```python
from build123d import *

# Parameters (mm, degrees)
SKETCH_1_W               = 90
SKETCH_1_H               = 48
EXTRUDE_1_DEPTH          = 8
SKETCH_4_R               = 15
CUT_EXTRUDE_3_DEPTH      = 3
SKETCH_5_R               = 1.8
CUT_EXTRUDE_4_DEPTH      = 3
MIRROR_2_COPY_1_SKETCH_R = 1.8
MIRROR_2_COPY_1_DEPTH    = 3
SKETCH_6_W               = 16
SKETCH_6_H               = 15
CUT_EXTRUDE_5_DEPTH      = 2.5


with BuildPart() as part:
    # 草图1 → 凸台-拉伸1 (new body)
    with BuildSketch(Plane.XY):
        Rectangle(SKETCH_1_W, SKETCH_1_H)
    extrude(amount=EXTRUDE_1_DEPTH)

    # 草图4 → 切除-拉伸3 (cut)
    with BuildSketch(Plane(origin=(0, 0, 0), x_dir=(-1, 0, 0), z_dir=(0, 0, -1))):
        Circle(SKETCH_4_R)
    extrude(amount=-CUT_EXTRUDE_3_DEPTH, mode=Mode.SUBTRACT)

    # 草图5 → 切除-拉伸4 (cut)
    with BuildSketch(Plane(origin=(0, 0, 0), x_dir=(-1, 0, 0), z_dir=(0, 0, -1))):
        with Locations((-41, 21)):
            Circle(SKETCH_5_R)
    cut_extrude_4 = extrude(amount=-CUT_EXTRUDE_4_DEPTH, mode=Mode.SUBTRACT)

    # 镜向1: 切除-拉伸4 across plane
    add(cut_extrude_4.mirror(Plane.ZX), mode=Mode.SUBTRACT)

    # 镜向2: 切除-拉伸4 across plane
    add(cut_extrude_4.mirror(Plane(origin=(0, 0, 0), x_dir=(0, 0, 1), z_dir=(1, 0, 0))), mode=Mode.SUBTRACT)

    # 镜向2 copy 1 sketch → 镜向2 copy 1 (cut)
    with BuildSketch(Plane(origin=(0, 0, 0), x_dir=(1, 0, 0), z_dir=(0, 0, -1))):
        with Locations((-41, 21)):
            Circle(MIRROR_2_COPY_1_SKETCH_R)
    extrude(amount=-MIRROR_2_COPY_1_DEPTH, mode=Mode.SUBTRACT)

    # 草图6 → 切除-拉伸5 (cut)
    with BuildSketch(Plane(origin=(0, 0, 0), x_dir=(-1, 0, 0), z_dir=(0, 0, -1))):
        with Locations((45, 0)):
            Rectangle(SKETCH_6_W, SKETCH_6_H)
    cut_extrude_5 = extrude(amount=-CUT_EXTRUDE_5_DEPTH, mode=Mode.SUBTRACT)

    # 镜向3: 切除-拉伸5 across plane
    add(cut_extrude_5.mirror(Plane(origin=(0, 0, 0), x_dir=(0, 0, 1), z_dir=(1, 0, 0))), mode=Mode.SUBTRACT)


solid = part.part
```
The model under review builds one solid part; all positions refer to its coordinate system, in mm. A direction names the side the tool comes from. Round coordinates to 2 decimals unless told otherwise and drop trailing zeros. Loops run counter-clockwise (first coordinate to the right, second up) from the corner with the lowest first, then second, coordinate; pieces in that order, holes last. Notation, with made-up numbers: M 46,42 L 50,42 A32 cw 50,71 Z; hole C -5.75,66 d3. An arc over 180 degrees is marked long. Put each result on its own line as item: value.
Q1. Consider section D-D, the plane y = -2.5. Give the boundary of the cut face in (x, z), then the cut area to 3 significant figures.
Result set:
outline: M -45,2.5 L -37,2.5 L -37,0 L -14.79,0 L -14.79,3 L 14.79,3 L 14.79,0 L 37,0 L 37,2.5 L 45,2.5 L 45,8 L -45,8 Z
area: 591 mm²
Q2. Machinability: for faces 4 (the flat face through (45, 0, 4)), 5 (the flat face through (-41, 0, 2.5)), 6 (the cylindrical face through (14.985, 0.66, 1.479)), 7 (the flat face through (37, 0, 1)), which of the approach directions +Z, -Z, +X, -X, +Y, -Y give a long, thin tool a straight path to every point of the face, cutting with its end or side? Answer none if there is none.
Result set:
face 4: +Z, -Z, +X, +Y, -Y
face 5: -Z, -X
face 6: -Z
face 7: -Z, +X
Q3. For pin 1 (3 mm diameter, centred on x = -41, y = -21, fed in from -Z), flat-tipped, find the tip position at first contact; note if it passes through.
Result set:
pin 1: stops at z = 3
Q4. Consider section B-B, the plane x = -9. Give the boundary of the cut face in (y, z).
Result set:
outline: M -24,0 L -12,0 L -12,3 L 12,3 L 12,0 L 24,0 L 24,8 L -24,8 Z
Q5. Mouldability with a two-part tool opening along Y and no side actions: class faces 1 (the flat face through (-1, 24, 4)), 2 (the cylindrical face through (40.032, -22.518, 1.479)), 3 (the flat face through (-11, 11, 0)) as released by +Y, released by -Y, zero draft, split by the parting line, or undercut.
Result set:
face 1: released by +Y
face 2: undercut
face 3: zero draft
Q6. Consider section C-C, the plane x = 0. Give the boundary of the cut face in (y, z).
Result set:
outline: M -24,0 L -15,0 L -15,3 L 15,3 L 15,0 L 24,0 L 24,8 L -24,8 Z
Q7. To check wall thickness, follow L1, parallel to Y at x = -41, z = 1.3; L2, parallel to X at y = -21, z = 0.95; L3, parallel to Y at x = 0, z = 1.1. State the ranges of each line that lie inside material, in increasing order.
Result set:
L1: y = -24 to -22.8, -19.2 to -7.5, 7.5 to 19.2, 22.8 to 24
L2: x = -45 to -42.8, -39.2 to 39.2, 42.8 to 45
L3: y = -24 to -15, 15 to 24
Q8. Consider section A-A, the plane y = -21. Give the boundary of the cut face in (x, z), then the cut area to 3 significant figures.
Result set:
outline: M -45,0 L -42.8,0 L -42.8,3 L -39.2,3 L -39.2,0 L 39.2,0 L 39.2,3 L 42.8,3 L 42.8,0 L 45,0 L 45,8 L -45,8 Z
area: 698 mm²
